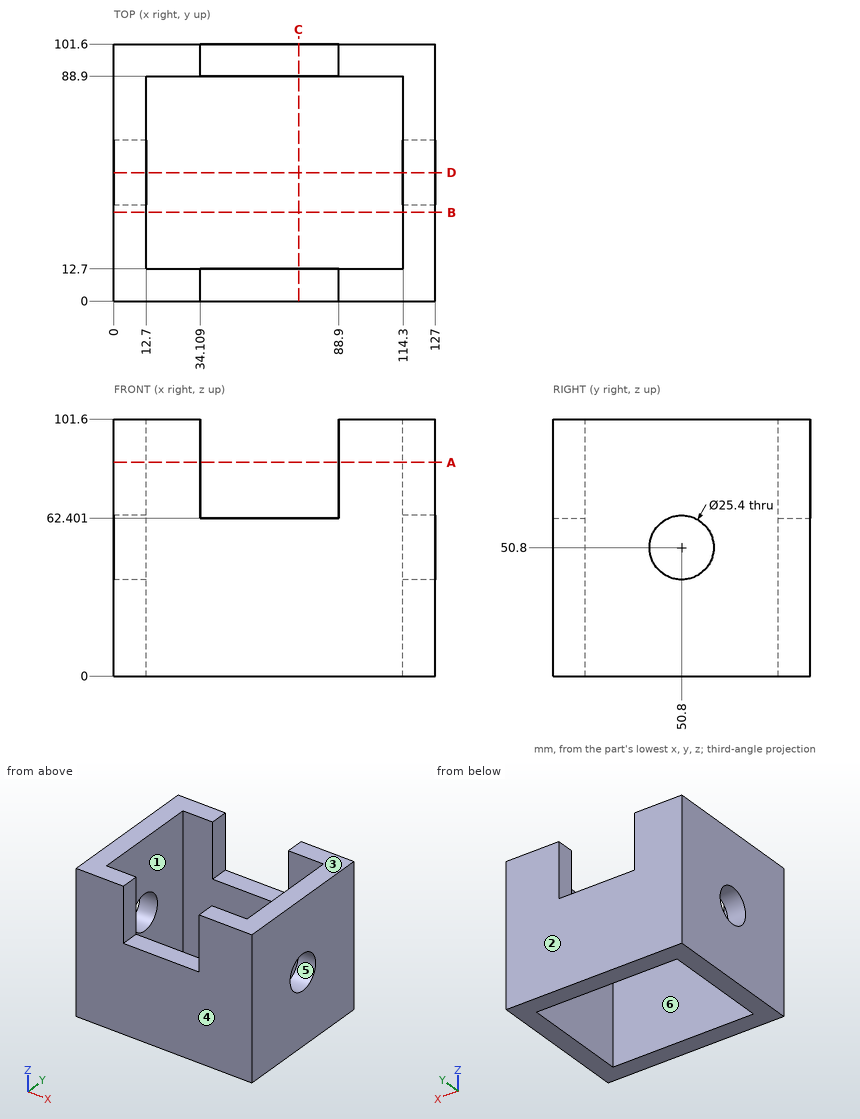
Geometry check sheet. Reference: drawing and pictorial views, mm from the part's lowest x, y, z. A direction names the side the tool comes from. Round coordinates to 2 decimals unless told otherwise and drop trailing zeros. Loops run counter-clockwise (first coordinate to the right, second up) from the corner with the lowest first, then second, coordinate; pieces in that order, holes last. Notation, with made-up numbers: (51, 12) -> (65, 12) arc R33 ccw to (65, 46) -> close; hole circle Ø10 at (22.5, 43). An arc over 180 degrees is marked (long way). Answer as a JSON object with one key per item and string values.
Q1. Section check C-C (x = 73). Record the boundary of the cut face in (y, z).
Data:
{"outline": "(0, 0) -> (12.7, 0) -> (12.7, 62.4) -> (0, 62.4) -> close; (88.9, 0) -> (101.6, 0) -> (101.6, 62.4) -> (88.9, 62.4) -> close"}
Q2. Access from +Z, -Z, +X, -X, +Y, -Y to the whole of each face (thin tool, end or side, straight path). Record for the marked faces 5 and 6.
Data:
{"face 5": "+X, -X", "face 6": "+Z, -Z"}
Q3. Go/stop test with flat-tipped pins: P1, Ø10, axis at x = 17, y = 73, coming from the +Z side; P2, Ø10, axis at x = 67, y = 4, coming from the +Z side; P3, Ø12, axis at x = 92.5, y = 20.5, coming from the +Z side. Record where each tip stops, or that it passes through.
Data:
{"P1": "stops at z = 101.6", "P2": "stops at z = 62.4", "P3": "passes through"}
Q4. Section check D-D (y = 50.8). Record the boundary of the cut face in (x, z).
Data:
{"outline": "(0, 0) -> (12.7, 0) -> (12.7, 38.1) -> (0, 38.1) -> close; (0, 63.5) -> (12.7, 63.5) -> (12.7, 101.6) -> (0, 101.6) -> close; (114.3, 0) -> (127, 0) -> (127, 38.1) -> (114.3, 38.1) -> close; (114.3, 63.5) -> (127, 63.5) -> (127, 101.6) -> (114.3, 101.6) -> close"}
Q5. Section check B-B (y = 35). Record the boundary of the cut face in (x, z).
Data:
{"outline": "(0, 0) -> (12.7, 0) -> (12.7, 101.6) -> (0, 101.6) -> close; (114.3, 0) -> (127, 0) -> (127, 101.6) -> (114.3, 101.6) -> close"}
Q6. Section check A-A (z = 84.5). Record the boundary of the cut face in (x, y), then the cut area to 3 significant figures.
Data:
{"outline": "(0, 0) -> (34.11, 0) -> (34.11, 12.7) -> (12.7, 12.7) -> (12.7, 88.9) -> (34.11, 88.9) -> (34.11, 101.6) -> (0, 101.6) -> close; (88.9, 0) -> (127, 0) -> (127, 101.6) -> (88.9, 101.6) -> (88.9, 88.9) -> (114.3, 88.9) -> (114.3, 12.7) -> (88.9, 12.7) -> close", "area": "3,770 mm2"}
Q7. Scan lines: line 1 (Y direction, x = 52, z = 40); line 2 (X direction, y = 65, z = 8); line 3 (Y direction, x = 4, z = 50) (1 decimal). Record each from-to range of solid material in increasing order. Write a range as from..to.
Data:
{"line 1": "y = 0..12.7, 88.9..101.6", "line 2": "x = 0..12.7, 114.3..127", "line 3": "y = 0..38.1, 63.5..101.6"}
Q8. Draft check along Y on the marked faces 1, 2, 3 and 4. Enter one of: pulls with the +Y half, pulls with the -Y half, needs draft (parallel to the pull), parting line crosses it, or undercut.
Data:
{"face 1": "undercut", "face 2": "pulls with the +Y half", "face 3": "needs draft", "face 4": "pulls with the -Y half"}
